from build123d import *

# Parameters (mm, degrees)
SKETCH_1_R          = 8.5
EXTRUDE_1_DEPTH     = 5
SKETCH_2_R          = 1.5
CUT_EXTRUDE_1_DEPTH = 5
CUT_EXTRUDE_2_DEPTH = 14.019216566
EXTRUDE_2_DEPTH     = 5
SKETCH_6_R          = 1.5
CUT_EXTRUDE_3_DEPTH = 22.759606561
FILLET_2_R          = 2


with BuildPart() as part:
    # 草图1 → 凸台-拉伸1 (new body)
    with BuildSketch(Plane.XY):
        Circle(SKETCH_1_R)
    extrude(amount=EXTRUDE_1_DEPTH)

    # 草图2 → 切除-拉伸1 (cut)
    with BuildSketch(Plane.XY.offset(5)):
        with Locations((0, 6.5)):
            Circle(SKETCH_2_R)
        with Locations((0, -6.5)):
            Circle(SKETCH_2_R)
    extrude(amount=-CUT_EXTRUDE_1_DEPTH, mode=Mode.SUBTRACT)

    # 草图3 → 切除-拉伸2 (cut, through all)
    with BuildSketch(Plane(origin=(0, 0, 0), x_dir=(-1, 0, 0), z_dir=(0, 0, -1))):
        with BuildLine():
            ThreePointArc((3.89097221, 2.724488073), (4.530155516, 1.428352548), (4.75, 0))
            Line((4.75, 0), (8.5, 0))
            ThreePointArc((8.5, 0), (8.106594081, 2.555999296), (6.962792376, 4.875399709))
            Line((6.962792376, 4.875399709), (3.89097221, 2.724488073))
        make_face()
        with BuildLine():
            Line((8.5, 0), (4.75, 0))
            ThreePointArc((4.75, 0), (4.530155516, -1.428352548), (3.89097221, -2.724488073))
            Line((3.89097221, -2.724488073), (6.962792376, -4.875399709))
            ThreePointArc((6.962792376, -4.875399709), (8.106594081, -2.555999296), (8.5, 0))
        make_face()
    cut_extrude_2 = extrude(amount=-CUT_EXTRUDE_2_DEPTH, mode=Mode.SUBTRACT)

    # 镜向1: 切除-拉伸2 across plane
    add(cut_extrude_2.mirror(Plane(origin=(0, 0, 0), x_dir=(0, 0, 1), z_dir=(1, 0, 0))), mode=Mode.SUBTRACT)


with BuildPart() as body_2:
    # 草图4 → 凸台-拉伸2 (new body)
    with BuildSketch(Plane(origin=(0, 0, 0), x_dir=(-1, 0, 0), z_dir=(0, 0, -1))):
        with BuildLine():
            ThreePointArc((6.962792376, -4.875399709), (0, -8.5), (-6.962792376, -4.875399709))
            Line((-6.962792376, -4.875399709), (-6.962792376, -20))
            Line((-6.962792376, -20), (6.962792376, -20))
            Line((6.962792376, -20), (6.962792376, -4.875399709))
        make_face()
    extrude(amount=-EXTRUDE_2_DEPTH)


with BuildPart() as part_1:
    add(part.part)

    # Combine 1: union body 2
    add(body_2.part)

    # 草图6 → 切除-拉伸3 (cut, through all)
    with BuildSketch(Plane(origin=(0, 0, 0), x_dir=(-1, 0, 0), z_dir=(0, 0, -1))):
        with BuildLine():
            Line((-6.962792376, 4.875399709), (-3.89097221, 2.724488073))
            Line((-3.89097221, 2.724488073), (-6.769757712, 5.140075925))
            ThreePointArc((-6.769757712, 5.140075925), (-6.867550244, 5.008667851), (-6.962792376, 4.875399709))
        make_face()
        with BuildLine():
            Line((-3.89097221, -2.724488073), (-3.89097221, 2.724488073))
            ThreePointArc((-3.89097221, 2.724488073), (-4.75, 0), (-3.89097221, -2.724488073))
        make_face()
        Polygon((-6.962792376, -5.302051241), (-3.89097221, -2.724488073), (-6.962792376, -4.875399709), align=None)
        with BuildLine():
            ThreePointArc((6.962792376, 4.875399709), (6.867550244, 5.008667851), (6.769757712, 5.140075925))
            Line((6.769757712, 5.140075925), (3.89097221, 2.724488073))
            Line((3.89097221, 2.724488073), (6.962792376, 4.875399709))
        make_face()
        with BuildLine():
            ThreePointArc((3.89097221, -2.724488073), (4.75, 0), (3.89097221, 2.724488073))
            Line((3.89097221, 2.724488073), (3.89097221, -2.724488073))
        make_face()
        Polygon((6.962792376, -4.875399709), (3.89097221, -2.724488073), (6.962792376, -5.302051241), align=None)
        Circle(SKETCH_6_R)
    extrude(amount=-CUT_EXTRUDE_3_DEPTH, mode=Mode.SUBTRACT)

    # 圆角2
    fillet_2_edges = [part_1.edges().sort_by_distance(p)[0] for p in [
        (-6.769757712, 5.140075925, 2.5),
        (6.769757712, 5.140075925, 2.5),
        (-3.89097221, -2.724488073, 2.5),
        (-3.89097221, 2.724488073, 2.5),
        (3.89097221, 2.724488073, 2.5),
        (3.89097221, -2.724488073, 2.5),
        (-6.962792376, -20, 2.5),
        (6.962792376, -20, 2.5),
        (6.962792376, -5.302051241, 2.5),
        (-6.962792376, -5.302051241, 2.5),
    ]]
    fillet(fillet_2_edges, radius=FILLET_2_R)


solid = part_1.part
The listing builds one solid part. Answer for the finished solid, in the listing's coordinates (mm). A direction names the side the tool comes from. Round coordinates to 2 decimals unless told otherwise and drop trailing zeros. Write each loop counter-clockwise with the first axis right and the second up, starting at its lowest first coordinate (ties: lowest second). Pieces come first, ordered by that corner, then holes. Notation, with made-up numbers: (32.5, 86.25) - (91.5, 86.25) arc R10 cw to (91.5, 92.25) - close; hole circle Ø5 at (45, 49). An arc over 180 degrees is marked (long way). Use a Markdown table: item, result. Add a question column.
1. For a pull along X with two mould halves and no side action, classify faces 1 (the face through (-6.77, -5.38, 2.54)), 2 (the face through (0, -8, 3)), 3 (the face through (4.084, -2.648, 2.535)) as +X half, -X half, draft (parallel to the pull), parting line (faces both ways), or undercut.
2. The part is cut by section C-C (x = -0.5). Write down the section's boundary in (y, z), and give its area (3 significant figures).
3. Flat-ended cylindrical pins translate along their axes: P1, Ø1.1, axis at y = 0, z = 3.5, coming from the +X side; P2, Ø1, axis at y = 0, z = 1, coming from the -X side. Find the tip coordinate at first contact, or state that the pin passes through.
4. The part is cut by section D-D (y = 0). Write down the section's boundary in (x, z), and give its area (3 significant figures).
5. Consider line 1 (Y direction, x = 0, z = 3.9); line 2 (X direction, y = 6, z = 3.75); line 3 (Y direction, x = 2.5, z = 0.75). Determine where each line is inside the solid, lowest interval first.
6. The part is cut by section A-A (y = -6.5). Write down the section's boundary in (x, z), and give its area (3 significant figures).
7. A tool of negligible diameter and unlimited length cuts with its end or side. For faces 4 (the face through (-4.084, 2.648, 2.535)), 5 (the face through (6.963, -12, 2)), 6 (the face through (4.073, 2.626, 2.535)), from which of +Z, -Z, +X, -X, +Y, -Y can it reach the whole face along a straight path? Write none if from no direction.
8. The part is cut by section B-B (z = 1.3). Write down the section's boundary in (x, y).
Reported:
| question | item | result |
|---|---|---|
| 1 | face 1 | -X half |
| 1 | face 2 | undercut |
| 1 | face 3 | +X half |
| 2 | outline | (-20, 0) - (-7.91, 0) - (-7.91, 5) - (-20, 5) - close; (-5.09, 0) - (-1.41, 0) - (-1.41, 5) - (-5.09, 5) - close; (1.41, 0) - (5.09, 0) - (5.09, 5) - (1.41, 5) - close; (7.91, 0) - (8.49, 0) - (8.49, 5) - (7.91, 5) - close |
| 2 | area | 100 mm^2 |
| 3 | P1 | x = 3.89 |
| 3 | P2 | x = -3.89 |
| 4 | outline | (-3.89, 0) - (-1.5, 0) - (-1.5, 5) - (-3.89, 5) - close; (1.5, 0) - (3.89, 0) - (3.89, 5) - (1.5, 5) - close |
| 4 | area | 23.9 mm^2 |
| 5 | line 1 | -20 to -8, -5 to -1.5, 1.5 to 5, 8 to 8.5 |
| 5 | line 2 | -5.67 to -1.41, 1.41 to 5.67 |
| 5 | line 3 | -20 to 8.12 |
| 6 | outline | (-6.96, 0) - (-1.5, 0) - (-1.5, 5) - (-6.96, 5) - close; (1.5, 0) - (6.96, 0) - (6.96, 5) - (1.5, 5) - close |
| 6 | area | 54.6 mm^2 |
| 7 | face 4 | +Z, -Z, -X |
| 7 | face 5 | +Z, -Z, +X, +Y, -Y |
| 7 | face 6 | +Z, -Z, +X |
| 8 | outline | (-6.96, -18) arc R2 ccw to (-4.96, -20) - (4.96, -20) arc R2 ccw to (6.96, -18) - (6.96, -6.23) arc R2 ccw to (6.25, -4.7) - (4.61, -3.32) arc R2 cw to (3.89, -1.79) - (3.89, 1.79) arc R2 cw to (4.61, 3.32) - (5.09, 3.73) arc R2 ccw to (4.98, 6.89) arc R8.5 ccw to (-4.98, 6.89) arc R2 ccw to (-5.09, 3.73) - (-4.61, 3.32) arc R2 cw to (-3.89, 1.79) - (-3.89, -1.79) arc R2 cw to (-4.61, -3.32) - (-6.25, -4.7) arc R2 ccw to (-6.96, -6.23) - close; hole circle Ø3 at (0, -6.5); hole circle Ø3 at (0, 0); hole circle Ø3 at (0, 6.5) |
